Could you check a few things on this model? Use its own coordinates, in mm. A direction names the side the tool comes from. Round coordinates to 2 decimals unless told otherwise and drop trailing zeros. Loops run counter-clockwise (first coordinate to the right, second up) from the corner with the lowest first, then second, coordinate; pieces in that order, holes last. Notation, with made-up numbers: M 70,60 L 80,60 A8 cw 80,68 Z; hole C 39,-18.5 d2. An arc over 180 degrees is marked long. Answer in a Markdown table with one row per item.
```python
from build123d import *

# Parameters (mm, degrees)
SKETCH1_W           = 9.525
SKETCH1_H           = 137.414
BOSS_EXTRUDE1_DEPTH = 63.5
SKETCH2_R           = 1.5875
CUT_EXTRUDE1_DEPTH  = 9.525


with BuildPart() as part:
    # Sketch1 → Boss-Extrude1 (new body)
    with BuildSketch(Plane.XY):
        Rectangle(SKETCH1_W, SKETCH1_H)
    extrude(amount=BOSS_EXTRUDE1_DEPTH)

    # Sketch2 → Cut-Extrude1 (cut)
    with BuildSketch(Plane(origin=(0, 68.707, 0), x_dir=(1, 0, 0), z_dir=(0, 1, 0))):
        with Locations(Location((0, -5.08, 0), (0, 0, 270))):
            Circle(SKETCH2_R)
        with Locations(Location((0, -31.75, 0), (0, 0, 270))):
            Circle(SKETCH2_R)
        with Locations(Location((0, -58.42, 0), (0, 0, 270))):
            Circle(SKETCH2_R)
    cut_extrude1 = extrude(amount=-CUT_EXTRUDE1_DEPTH, mode=Mode.SUBTRACT)

    # Mirror1: Cut-Extrude1 across plane
    add(cut_extrude1.mirror(Plane.ZX), mode=Mode.SUBTRACT)


solid = part.part
```
1) If we mould it in two halves opening along X, with no side actions, what happens to faces 4 (the face through (0.477, 64.011, 6.594)), 5 (the face through (-4.762, -1, 31)), 6 (the face through (2, 68.707, 31))? For each: released by +X, released by -X, zero draft, split by the parting line, or undercut.
Computed:
| item | result |
|---|---|
| face 4 | undercut |
| face 5 | released by -X |
| face 6 | zero draft |
2) I want a section at B-B, the plane z = 58.42. Please give me the cut outline in (x, y).
Computed:
| item | result |
|---|---|
| outline | M -4.76,-68.71 L -1.59,-68.71 L -1.59,-59.18 L 1.59,-59.18 L 1.59,-68.71 L 4.76,-68.71 L 4.76,68.71 L 1.59,68.71 L 1.59,59.18 L -1.59,59.18 L -1.59,68.71 L -4.76,68.71 Z |
3) Will these pins go through, and if not, where does the flat tip stop? P1, Ø4, axis at x = 0, z = 58.42, coming from the +Y side; P2, Ø1.6, axis at x = 0, z = 5.5, coming from the -Y side; P3, Ø2.5, axis at x = 0, z = 58.42, coming from the +Y side.
Computed:
| item | result |
|---|---|
| P1 | stops at y = 68.71 |
| P2 | stops at y = -59.18 |
| P3 | stops at y = 59.18 |
4) I want a section at A-A, the plane x = 0. Please give me the cut outline in (y, z).
Computed:
| item | result |
|---|---|
| outline | M -68.71,0 L 68.71,0 L 68.71,3.49 L 59.18,3.49 L 59.18,6.67 L 68.71,6.67 L 68.71,30.16 L 59.18,30.16 L 59.18,33.34 L 68.71,33.34 L 68.71,56.83 L 59.18,56.83 L 59.18,60.01 L 68.71,60.01 L 68.71,63.5 L -68.71,63.5 L -68.71,60.01 L -59.18,60.01 L -59.18,56.83 L -68.71,56.83 L -68.71,33.34 L -59.18,33.34 L -59.18,30.16 L -68.71,30.16 L -68.71,6.67 L -59.18,6.67 L -59.18,3.49 L -68.71,3.49 Z |
5) Which directions (+Z, -Z, +X, -X, +Y, -Y) give clear straight access to the entire face, cutting with the end or side of a thin tool? Please do faces 1 (the face through (0.477, 64.011, 33.264)), 2 (the face through (0, 1, 63.5)), 3 (the face through (0, -59.182, 5)).
Computed:
| item | result |
|---|---|
| face 1 | +Y |
| face 2 | +Z, +X, -X, +Y, -Y |
| face 3 | -Y |
6) I need wall thicknesses on line 1 (X direction, y = 65, z = 5); line 2 (Y direction, x = -0.25, z = 31); line 3 (X direction, y = -66, z = 31). Which ranges of each line are inside material? Lowest first, please.
Computed:
| item | result |
|---|---|
| line 1 | x = -4.76 to -1.59, 1.59 to 4.76 |
| line 2 | y = -59.18 to 59.18 |
| line 3 | x = -4.76 to -1.4, 1.4 to 4.76 |
